Geometry: final body of the model. Coordinates: model frame, mm. A direction names the side the tool comes from. Coordinates: 2 decimals unless noted, no trailing zeros. Loops run counter-clockwise (first coordinate to the right, second up) from the corner with the lowest first, then second, coordinate; pieces in that order, holes last. Notation, with made-up numbers: (-1, 56.25) - (11, 56.25) arc R28 ccw to (11, 84.25) - close; hole circle Ø2 at (77, 43). An arc over 180 degrees is marked (long way). Return JSON: item names as keys, results as strings.
from build123d import *

# Parameters (mm, degrees)
F0_W     = 160
F0_H     = 60
F1_DEPTH = 15
F2_R     = 3
F3_T     = -2.5
F5_DEPTH = 10
F6_W     = 85
F6_H     = 25
F7_DEPTH = 25


with BuildPart() as f1:
    # F0 (on Front) → F1 (new body)
    with BuildSketch(Plane.XZ):
        with Locations((80, 30)):
            Rectangle(F0_W, F0_H)
    extrude(amount=F1_DEPTH)

    # F2
    f2_edges = [f1.edges().sort_by_distance(p)[0] for p in [
        (0, -7.5, 60),
        (80, -15, 60),
        (0, -15, 30),
        (80, -15, 0),
        (0, -7.5, 0),
        (160, -7.5, 0),
        (160, -7.5, 60),
        (160, -15, 30),
    ]]
    fillet(f2_edges, radius=F2_R)

    # F3
    f3_openings = [f1.faces().sort_by_distance(p)[0] for p in [
        (80, 0, 30),
    ]]
    offset(amount=F3_T, openings=f3_openings)

    # F4 (on face) → F5 (join)
    with BuildSketch(Plane(origin=(0, -12.5, 0), x_dir=(-1, 0, 0), z_dir=(0, 1, 0))):
        with BuildLine():
            ThreePointArc((-157, 50.417424305), (-152.2613872125, 50.8166998673), (-150, 55))
            ThreePointArc((-150, 55), (-150.1054684353, 56.0215482184), (-150.417424305, 57))
            Line((-150.417424305, 57), (-157, 57))
            Line((-157, 57), (-157, 50.417424305))
        make_face()
        with BuildLine():
            Line((-3, 57), (-9.582575695, 57))
            ThreePointArc((-9.582575695, 57), (-8.5355339059, 51.4644660941), (-3, 50.417424305))
            Line((-3, 50.417424305), (-3, 57))
        make_face()
        with BuildLine():
            ThreePointArc((-150, 5), (-152.2613872125, 9.1833001327), (-157, 9.582575695))
            Line((-157, 9.582575695), (-157, 3))
            Line((-157, 3), (-150.417424305, 3))
            ThreePointArc((-150.417424305, 3), (-150.1054684353, 3.9784517816), (-150, 5))
        make_face()
        with BuildLine():
            Line((-3, 3), (-3, 9.582575695))
            ThreePointArc((-3, 9.582575695), (-8.5355339059, 8.5355339059), (-9.582575695, 3))
            Line((-9.582575695, 3), (-3, 3))
        make_face()
    extrude(amount=F5_DEPTH)

    # F6 (on face) → F7 (cut)
    with BuildSketch(Plane(origin=(0, -12.5, 0), x_dir=(-1, 0, 0), z_dir=(0, 1, 0))):
        with Locations((-87.5, 30)):
            Rectangle(F6_W, F6_H)
    extrude(amount=-F7_DEPTH, mode=Mode.SUBTRACT)


solid = f1.part
Item 1: Ray query, probe 1 along Z at (x, y) = (126, -8.5); probe 2 along X at (y, z) = (-10.5, 28.5); probe 3 along Z at (x, y) = (9, -7.5). Return the intervals inside material, ascending. Write a range as from..to.
Worked out:
{"probe 1": "0..2.5, 57.5..60", "probe 2": "0..2.5, 157.5..160", "probe 3": "0..2.5, 3..8, 52..57, 57.5..60"}
Item 2: Section query D-D, the plane z = 16. Return loops of the section in (x, y), and give its area (3 significant figures).
Worked out:
{"outline": "(0, -12) arc R3 ccw to (3, -15) - (157, -15) arc R3 ccw to (160, -12) - (160, 0) - (157.5, 0) - (157.5, -12) arc R0.5 cw to (157, -12.5) - (3, -12.5) arc R0.5 cw to (2.5, -12) - (2.5, 0) - (0, 0) - close", "area": "459 mm^2"}
Item 3: First-contact query: pin 1 Ø7.5 at (x, z) = (152, 52.5) entering from +Y; pin 2 Ø2 at (x, z) = (102.5, 16.5) entering from +Y; pin 3 Ø0.8 at (x, y) = (68.5, -14) entering from -Z. Flat tips, straight axial feed; report the tip coordinate or a pass-through.
Worked out:
{"pin 1": "y = -2.5", "pin 2": "y = -12.5", "pin 3": "z = 0.46"}
Item 4: Mould query, pull axis X, two halves, no side actions, for faces 3 (the face through (81.08, -14.1, 0.86)), 4 (the face through (0.86, -6.08, 59.1)), 5 (the face through (6, -8, 57)). Classes: +X half, -X half, draft (parallel to the pull), parting line (faces both ways), or undercut.
Worked out:
{"face 3": "draft", "face 4": "-X half", "face 5": "undercut"}
Item 5: Reachability of faces 1 (the face through (80, 0, 1)), 2 (the face through (154, -2.5, 54)) from +Z, -Z, +X, -X, +Y, -Y: full face, straight path, thin tool, end or side. Return the list, or none.
Worked out:
{"face 1": "+Z, -Z, +X, -X, +Y", "face 2": "+Y"}
Item 6: Section query B-B, the plane x = 100. Return loops of the section in (y, z).
Worked out:
{"outline": "(-15, 3) arc R3 ccw to (-12, 0) - (0, 0) - (0, 2.5) - (-12, 2.5) arc R0.5 cw to (-12.5, 3) - (-12.5, 17.5) - (-15, 17.5) - close; (-15, 42.5) - (-12.5, 42.5) - (-12.5, 57) arc R0.5 cw to (-12, 57.5) - (0, 57.5) - (0, 60) - (-12, 60) arc R3 ccw to (-15, 57) - close"}
Item 7: Section query C-C, the plane z = 23.5. Return loops of the section in (x, y).
Worked out:
{"outline": "(0, -12) arc R3 ccw to (3, -15) - (45, -15) - (45, -12.5) - (3, -12.5) arc R0.5 cw to (2.5, -12) - (2.5, 0) - (0, 0) - close; (130, -15) - (157, -15) arc R3 ccw to (160, -12) - (160, 0) - (157.5, 0) - (157.5, -12) arc R0.5 cw to (157, -12.5) - (130, -12.5) - close"}
Item 8: Section query A-A, the plane y = -5. Return loops of the section in (x, z).
Worked out:
{"outline": "(0, 3) arc R3 ccw to (3, 0) - (157, 0) arc R3 ccw to (160, 3) - (160, 57) arc R3 ccw to (157, 60) - (3, 60) arc R3 ccw to (0, 57) - close; (3, 3) - (9.58, 3) arc R5 ccw to (3, 9.58) - close; (3, 50.42) arc R5 ccw to (9.58, 57) - (3, 57) - close; (150.42, 3) - (157, 3) - (157, 9.58) arc R5 ccw to start; (150.42, 57) arc R5 ccw to (157, 50.42) - (157, 57) - close; hole (2.5, 3) arc R0.5 ccw to (3, 2.5) - (157, 2.5) arc R0.5 ccw to (157.5, 3) - (157.5, 57) arc R0.5 ccw to (157, 57.5) - (3, 57.5) arc R0.5 ccw to (2.5, 57) - close"}
